from build123d import *

# Parameters (mm, degrees)
F1_DEPTH = 2
F2_R     = 5.025
F3_DEPTH = 1.65


with BuildPart() as f1:
    # F0 (on Front) → F1 (new body)
    with BuildSketch(Plane.XZ):
        with BuildLine():
            ThreePointArc((0, 7), (2.050253, 2.050253), (7, 0))
            Line((7, 0), (143, 0))
            ThreePointArc((143, 0), (147.949747, 2.050253), (150, 7))
            Line((150, 7), (150, 23))
            ThreePointArc((150, 23), (147.949747, 27.949747), (143, 30))
            Line((143, 30), (7, 30))
            ThreePointArc((7, 30), (2.050253, 27.949747), (0, 23))
            Line((0, 23), (0, 7))
        make_face()
    extrude(amount=F1_DEPTH)

    # F2 (on face) → F3 (cut)
    with BuildSketch(Plane.XZ.offset(2)):
        with Locations((20, 15)):
            Circle(F2_R)
        with Locations((47.5, 15)):
            Circle(F2_R)
        with Locations((75, 15)):
            Circle(F2_R)
        with Locations((102.5, 15)):
            Circle(F2_R)
        with Locations((130, 15)):
            Circle(F2_R)
    extrude(amount=-F3_DEPTH, mode=Mode.SUBTRACT)


solid = f1.part
Geometry: final body of the model. Coordinates: model frame, mm. A direction names the side the tool comes from. Round coordinates to 2 decimals unless told otherwise and drop trailing zeros. Loops run counter-clockwise (first coordinate to the right, second up) from the corner with the lowest first, then second, coordinate; pieces in that order, holes last. Notation, with made-up numbers: M 10.25,52 L 17.25,52 A34 ccw 17.25,87 Z; hole C 42,6 d4. An arc over 180 degrees is marked long. Put each result on its own line as item: value. Start each with the question number.
(1) Contact query for a flat-ended pin moving along its axis: pin 1 Ø3 at (x, z) = (76, 13) entering from -Y. Output: stop coordinate, or through.
(2) Section query C-C (z = 15). Return loops of the section in (x, y) (3 decimals), then the cut area to 3 significant figures.
(3) Set-up query: faces 5 (the face through (47, -0.35, 15)), 6 (the face through (147.9, -1, 2)). Return all of +Z, -Z, +X, -X, +Y, -Y with unobstructed straight access to the full face (end or side cutting, diameter ignored); none if empty.
(4) Section query D-D (x = 102). Return loops of the section in (y, z).
(5) Material intervals for line 1 along Z through (x, y) = (20, -0.9) (3 decimals); line 2 along X through (y, z) = (-1.7, 13.5); line 3 along Y through (x, z) = (75, 10.5), sorted ascending. Write a range as [from, to].
(6) Section query A-A (y = -0.8). Return loops of the section in (x, z) (3 decimals).
(7) Section query B-B (x = 20). Return loops of the section in (y, z) (3 decimals).
(8) Draft query along X for faces 1 (the face through (98.8, -1.2, 18.4)), 2 (the face through (148, -1, 27.9)), 3 (the face through (71.3, -1.2, 18.4)), 4 (the face through (74, -2, 9)). Return one class per face: +X half, -X half, draft (parallel to the pull), parting line (faces both ways), or undercut.
Findings below:
1. pin 1: stops at y = -0.35
2. outline: M 0,-2 L 14.975,-2 L 14.975,-0.35 L 25.025,-0.35 L 25.025,-2 L 42.475,-2 L 42.475,-0.35 L 52.525,-0.35 L 52.525,-2 L 69.975,-2 L 69.975,-0.35 L 80.025,-0.35 L 80.025,-2 L 97.475,-2 L 97.475,-0.35 L 107.525,-0.35 L 107.525,-2 L 124.975,-2 L 124.975,-0.35 L 135.025,-0.35 L 135.025,-2 L 150,-2 L 150,0 L 0,0 Z
2. area: 217 mm2
3. face 5: -Y
3. face 6: -Z, +X, +Y, -Y
4. outline: M -2,0 L 0,0 L 0,30 L -2,30 L -2,20 L -0.35,20 L -0.35,10 L -2,10 Z
5. line 1: z = [0, 9.975], [20.025, 30]
5. line 2: x = [0, 15.2], [24.8, 42.7], [52.3, 70.2], [79.8, 97.7], [107.3, 125.2], [134.8, 150]
5. line 3: y = [-0.35, 0]
6. outline: M 0,7 A7 ccw 7,0 L 143,0 A7 ccw 150,7 L 150,23 A7 ccw 143,30 L 7,30 A7 ccw 0,23 Z; hole C 20,15 d10.05; hole C 47.5,15 d10.05; hole C 75,15 d10.05; hole C 102.5,15 d10.05; hole C 130,15 d10.05
7. outline: M -2,0 L 0,0 L 0,30 L -2,30 L -2,20.025 L -0.35,20.025 L -0.35,9.975 L -2,9.975 Z
8. face 1: undercut
8. face 2: +X half
8. face 3: undercut
8. face 4: draft
